Autodesk Inventor part; units mm, degrees
ref_plane "YZ Plane" through (0, 0, 0) normal (1, 0, 0) x (0, 1, 0)
ref_plane "XZ Plane" through (0, 0, 0) normal (0, 1, 0) x (-1, 0, 0)
sketch "Skizze1" plane through (0, 0, 0) normal (0, 1, 0) x (-1, 0, 0)
  line L0 (0, -20) -> (33.5, -20)
  line L1 (33.5, -20) -> (33.5, 18)
  line L2 (33.5, 18) -> (0, 18)
  line L3 (0, 18) -> (0, -20)
  line L4 (-6.7, 0) -> (40.2, 0)
  line L5 (0, 18) -> (0, 20.5)
  line L6 (0, 20.5) -> (8.5, 20.5)
  line L7 (8.5, 20.5) -> (8.5, 18)
  line L8 (25, 12) -> (8.5, 12)
  line L9 (8.5, 12) -> (8.5, -16)
  line L10 (8.5, -16) -> (25, -16)
  line L11 (25, -16) -> (25, 12)
  point P0 (0, 0)
  dimension "d1" = 33.5
  dimension "d4" = 18
  dimension "d5" = 20
  dimension "d6" = 2.5
  dimension "d7" = 8.5
  dimension "d8" = 6
  dimension "d9" = 4
  dimension "d10" = 8.5
  dimension "d11" = 8.5
extrude "Extrusion1" add sketch "Skizze1" along normal blind 1.5 contours L3 L4 L9 L10 L11 L1 L0 | L3 L2 L1 L4 L11 L8 L9 | L5 L6 L7 L2
sketch "Skizze2" plane through (-8.5, 0, -16) normal (-1, 0, 0) x (0, 0, 1)
  line L0 (28, 0) -> (0, 0)
  line L1 (17.6, 0) -> (17.6, -5.5)
  line L2 (17.6, -5.5) -> (18.6, -5.5)
  line L3 (18.6, -5.5) -> (18.6, 0)
  line L4 (21, 0) -> (21, -5.5)
  line L5 (21, -5.5) -> (22, -5.5)
  line L6 (22, -5.5) -> (22, 0)
  line L7 (16, 2.6) -> (16, -5.1)
  line L8 (21, -4) -> (18.6, -4)
  line L9 (17.6, -5.5) -> (0, 0)
  point P0 (16, 0)
  point P1 (16, -5)
  dimension "d12" = 2.6
  dimension "d13" = 5
  dimension "d14" = 1
  dimension "d15" = 1
  dimension "d16" = 5.5
  dimension "d19" = 4
extrude "Extrusion2" add sketch "Skizze2" against normal blind 1.5
sketch "Skizze3" plane through (-8.5, 0, 12) normal (-1, 0, 0) x (0, 0, 1)
  line L0 (-32, 1.5) -> (6, 1.5)
  line L1 (-6, -5.5) -> (-6, 0)
  line L2 (-6, 0) -> (-28, 0)
  line L3 (-6, 0) -> (-6, 1.5)
  line L4 (-6, 0) -> (-6, -5.5)
  line L5 (-6, -3) -> (-11, -3)
  line L6 (-11, -3) -> (-23, 1.5)
  line L7 (8.5, 1.5) -> (-32, 1.5)
  line L8 (-9.4, -4) -> (-7, -4)
  line L9 (-28, 0) -> (-28, 1.5)
  point P0 (-12, 0)
  dimension "d20" = 1
  dimension "d21" = 5
  dimension "d23" = 5
extrude "Extrusion3" cut sketch "Skizze3" against normal up to surface (1.5 mm away) contours L0 L3 L2 L6 | L2 L1 L5 L6
sketch "Skizze4" plane through (-33.5, 0, -20) normal (-1, 0, 0) x (0, 0, 1)
  line L0 (32, 0) -> (4, 0)
  line L1 (16, 0) -> (16, -12)
  line L2 (16, -12) -> (17, -12)
  line L3 (17, -12) -> (17.8, -4)
  line L4 (17.8, -4) -> (20, -4)
  line L5 (20, -4) -> (20, 0)
  line L6 (20, 5.3565) -> (20, -21.6388)
  dimension "d26" = 3
  dimension "d27" = 2.2
  dimension "d28" = 4
  dimension "d29" = 8
  dimension "d30" = 12
extrude "Extrusion4" add sketch "Skizze4" against normal blind 2
mirror "Spiegeln1" about plane through (0, 0, 0) normal (0, 0, 1) of "Extrusion4"
sketch "Skizze5" plane through (0, 1.5, 0) normal (0, 1, 0) x (1, 0, 0)
  line L0 (6.7, 0) -> (-40.2, 0)
  line L1 (0, -20.5) -> (0, 20)
  point P0 (0, 0)
  point P1 (-29.25, -13.45)
  point P2 (-29.25, 13.45)
  point P3 (-4.25, -15.8)
  point P4 (-4.25, 19.9)
  dimension "d33" = 13.45
  dimension "d34" = 13.45
  dimension "d35" = 15.8
  dimension "d36" = 19.9
  dimension "d37" = 4.25
  dimension "d38" = 29.25
hole "Bohrung1" at (-29.25, 1.5, 13.45) at (-29.25, 1.5, -13.45) at (-4.25, 1.5, 15.8) at (-4.25, 1.5, -19.9) direction (0, -1, 0) diameter 3.4 depth 23.75 tip angle 118
properties part number "servo_und_kabelhalter"
Here's how the part is built. I have some questions about the finished solid (model axes, mm). A direction names the side the tool comes from. Coordinates: 2 decimals unless noted, no trailing zeros. Loops run counter-clockwise (first coordinate to the right, second up) from the corner with the lowest first, then second, coordinate; pieces in that order, holes last. Notation, with made-up numbers: (20, 32.5) -> (48, 32.5) arc R6 cw to (48, 36.5) -> close; hole circle Ø5 at (-32, 37). An arc over 180 degrees is marked (long way). Return JSON: item names as keys, results as strings.
1) I need wall thicknesses on line 1 (Z direction, x = -29.25, y = 1.1); line 2 (X direction, y = 0.5, z = -13.45); line 3 (X direction, y = 1.15, z = 13.45). Which ranges of each line are inside material? Lowest first, please. Write a range as from..to.
Results below:
{"line 1": "-20..-15.15, -11.75..11.75, 15.15..18", "line 2": "-33.5..-30.95, -27.55..-25, -8.5..0", "line 3": "-33.5..-30.95, -27.55..0"}
2) If we section it at C-C, the plane y = -9: Write out the boundary of the cut face in (x, z).
Results below:
{"outline": "(-33.5, -4) -> (-31.5, -4) -> (-31.5, -2.7) -> (-33.5, -2.7) -> close; (-33.5, 2.7) -> (-31.5, 2.7) -> (-31.5, 4) -> (-33.5, 4) -> close"}
3) Will these pins go through, and if not, where does the flat tip stop? pin 1 (5 mm diameter, centred on y = -3, z = 2.5, fed in from +X); pin 2 (1.6 mm diameter, centred on x = -32.5, y = -4.5, fed in from -Z); pin 3 (1 mm diameter, centred on y = -8, z = -3.5, fed in from +X); pin 4 (1.5 mm diameter, centred on x = -25, y = -1, fed in from +Z).
Results below:
{"pin 1": "x = -7", "pin 2": "z = -4", "pin 3": "x = -31.5", "pin 4": "through"}
4) If we section it at A-A, the plane z = 4.5: Write out the boundary of the cut face in (x, y), then the cut area to 4 significant figures.
Results below:
{"outline": "(-33.5, 0) -> (-25, 0) -> (-25, 1.5) -> (-33.5, 1.5) -> close; (-8.5, -4) -> (-7, -4) -> (-7, -3) -> (-8.5, -3) -> close; (-7, 0) -> (0, 0) -> (0, 1.5) -> (-7, 1.5) -> close", "area": "24.75 mm²"}
5) If we section it at B-B, the plane x = -12: Write out the boundary of the cut face in (y, z).
Results below:
{"outline": "(0, -20) -> (1.5, -20) -> (1.5, -16) -> (0, -16) -> close; (0, 12) -> (1.5, 12) -> (1.5, 18) -> (0, 18) -> close"}
6) If we section it at D-D, the plane x = -29.25: Write out the boundary of the cut face in (y, z), then the cut area to 3 significant figures.
Results below:
{"outline": "(0, -20) -> (1.5, -20) -> (1.5, -15.15) -> (0, -15.15) -> close; (0, -11.75) -> (1.5, -11.75) -> (1.5, 11.75) -> (0, 11.75) -> close; (0, 15.15) -> (1.5, 15.15) -> (1.5, 18) -> (0, 18) -> close", "area": "46.8 mm²"}
7) Thinking about a two-plate mould opening in X: for faces 1 (the face through (-8, 1, 6)), 2 (the face through (-33.5, -2, -1)), 3 (the face through (-32.5, -12, -3.5)), which applies, +X half, -X half, draft (parallel to the pull), parting line (faces both ways), or undercut?
Results below:
{"face 1": "undercut", "face 2": "-X half", "face 3": "draft"}
8) For faces 4 (the face through (-8, -4, 4)), 5 (the face through (-17, 1, -16)), 6 (the face through (-33, -6, -4)), which set-ups out of +Z, -Z, +X, -X, +Y, -Y let a thin tool reach every point of the face, with its end or its side?
Results below:
{"face 4": "+X, -Y", "face 5": "+Y, -Y", "face 6": "-Z, -X, -Y"}
